Here's how the part is built. I have some questions about the finished solid (model axes, mm). Face numbers are marked on the shaded views. A direction names the side the tool comes from. Coordinates: 2 decimals unless noted, no trailing zeros. Write each loop counter-clockwise with the first axis right and the second up, starting at its lowest first coordinate (ties: lowest second). Pieces come first, ordered by that corner, then holes. Notation, with made-up numbers: (-12.75, 34) - (0.25, 34) arc R22 ccw to (0.25, 73) - close; hole circle Ø8 at (-9, -38.5). An arc over 180 degrees is marked (long way). Answer in a Markdown table with one row per item. Add a question column.
Item 1: Imagine slicing it at D-D (z = 29). Please give me the cut outline in (x, y).
Item 2: We'd pull the mould along X, two halves only. Please class the marked faces 3, 4 and 5: +X half, -X half, draft (parallel to the pull), parting line (faces both ways), or undercut.
Item 3: If I drill on probe 1 along X at (y, z) = (-16, 54); probe 2 along Z at (x, y) = (30.15, 0); probe 3 along Y at (x, z) = (20.5, 16.5), over which ranges is the centre line in solid material (lowest first)? Write a range as from..to.
Item 4: Imagine slicing it at B-B (x = -13.5). Please give me the cut outline in (y, z).
Item 5: Imagine slicing it at C-C (y = 0). Please give me the cut outline in (x, z).
Item 6: I'm going to push a flat-ended pin straight in: pin 1 (18 mm diameter, centred on y = 0, z = 31.75, fed in from -X). Where does the tip first touch, or does it pass through?
Item 7: Which directions (+Z, -Z, +X, -X, +Y, -Y) give clear straight access to the entire face, cutting with the end or side of a thin tool? Please do the marked faces 1 and 2.
Item 8: Imagine slicing it at A-A (y = -17). Please give me the cut outline in (x, z), plus the area to 3 significant figures.
from build123d import *

# Parameters (mm, degrees)
F0_W     = 63.5
F0_H     = 63.5
F0_W_2   = 57.5
F0_H_2   = 57.5
F1_DEPTH = 63.5
F2_R     = 15
F3_DEPTH = 3
F4_R     = 15
F5_DEPTH = 3


with BuildPart() as f1:
    # F0 (on Top) → F1 (new body)
    with BuildSketch(Plane.XY):
        with Locations((0.304607, 0.271222)):
            Rectangle(F0_W, F0_H)
        with Locations((0.304607, 0.271222)):
            Rectangle(F0_W_2, F0_H_2, mode=Mode.SUBTRACT)
    extrude(amount=F1_DEPTH)

    # F2 (on face) → F3 (cut)
    with BuildSketch(Plane.YZ.offset(32.054607)):
        with Locations((0, 31.75)):
            Circle(F2_R)
    extrude(amount=-F3_DEPTH, mode=Mode.SUBTRACT)

    # F4 (on face) → F5 (cut)
    with BuildSketch(Plane(origin=(-31.445393, 0, 0), x_dir=(0, -1, 0), z_dir=(-1, 0, 0))):
        with Locations((0, 31.75)):
            Circle(F4_R)
    extrude(amount=-F5_DEPTH, mode=Mode.SUBTRACT)


solid = f1.part
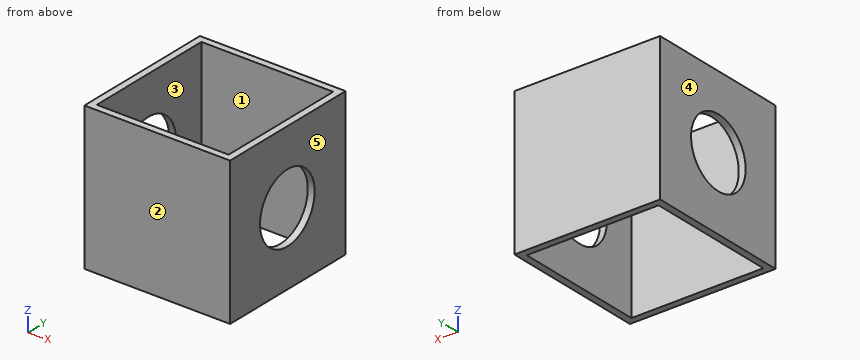
Here are the results:
| question | item | result |
|---|---|---|
| 1 | outline | (-31.45, -31.48) - (32.05, -31.48) - (32.05, -14.75) - (29.05, -14.75) - (29.05, -28.48) - (-28.45, -28.48) - (-28.45, -14.75) - (-31.45, -14.75) - close; (-31.45, 14.75) - (-28.45, 14.75) - (-28.45, 29.02) - (29.05, 29.02) - (29.05, 14.75) - (32.05, 14.75) - (32.05, 32.02) - (-31.45, 32.02) - close |
| 2 | face 3 | undercut |
| 2 | face 4 | -X half |
| 2 | face 5 | +X half |
| 3 | probe 1 | x = -31.45..-28.45, 29.05..32.05 |
| 3 | probe 2 | z = 0..16.75, 46.75..63.5 |
| 3 | probe 3 | y = -31.48..-28.48, 29.02..32.02 |
| 4 | outline | (-31.48, 0) - (-28.48, 0) - (-28.48, 63.5) - (-31.48, 63.5) - close; (29.02, 0) - (32.02, 0) - (32.02, 63.5) - (29.02, 63.5) - close |
| 5 | outline | (-31.45, 0) - (-28.45, 0) - (-28.45, 16.75) - (-31.45, 16.75) - close; (-31.45, 46.75) - (-28.45, 46.75) - (-28.45, 63.5) - (-31.45, 63.5) - close; (29.05, 0) - (32.05, 0) - (32.05, 16.75) - (29.05, 16.75) - close; (29.05, 46.75) - (32.05, 46.75) - (32.05, 63.5) - (29.05, 63.5) - close |
| 6 | pin 1 | passes through |
| 7 | face 1 | +Z, -Z |
| 7 | face 2 | +Z, -Z, +X, -X, -Y |
| 8 | outline | (-31.45, 0) - (-28.45, 0) - (-28.45, 63.5) - (-31.45, 63.5) - close; (29.05, 0) - (32.05, 0) - (32.05, 63.5) - (29.05, 63.5) - close |
| 8 | area | 381 mm2 |
